from build123d import *

# Parameters (mm, degrees)
SKETCH_1_R          = 21.5
EXTRUDE_1_DEPTH     = 10
EXTRUDE_2_DEPTH     = 5
EXTRUDE_3_DEPTH     = 5
FILLET_1_R          = 10
SKETCH_4_R          = 25
CUT_EXTRUDE_1_DEPTH = 110.56761611
SKETCH_5_R          = 1.65
CUT_EXTRUDE_2_DEPTH = 110.56761611
SKETCH_6_R          = 2.15
CUT_EXTRUDE_3_DEPTH = 92.256849058


with BuildPart() as part:
    # ｽｹｯﾁ1 → ﾎﾞｽ - 押し出し1 (new body)
    with BuildSketch(Plane.XY):
        Circle(SKETCH_1_R)
    extrude(amount=EXTRUDE_1_DEPTH)

    # ｽｹｯﾁ2 → ﾎﾞｽ - 押し出し2 (add)
    with BuildSketch(Plane.XY.offset(10)):
        with BuildLine():
            Line((-21.5, 0), (-21.5, -25))
            Line((-21.5, -25), (21.5, -25))
            Line((21.5, -25), (21.5, 0))
            ThreePointArc((21.5, 0), (0, 21.5), (-21.5, 0))
        make_face()
    extrude(amount=EXTRUDE_2_DEPTH)

    # ｽｹｯﾁ3 → ﾎﾞｽ - 押し出し3 (add)
    with BuildSketch(Plane.XZ.offset(25)):
        with BuildLine():
            Line((-39.25, 54.25), (-39.25, 15))
            Line((-39.25, 15), (39.25, 15))
            Line((39.25, 15), (39.25, 54.25))
            ThreePointArc((39.25, 54.25), (0, 93.5), (-39.25, 54.25))
        make_face()
    extrude(amount=-EXTRUDE_3_DEPTH)

    # ﾌｨﾚｯﾄ1
    fillet_1_edges = [part.edges().sort_by_distance(p)[0] for p in [
        (39.25, -22.5, 15),
        (-39.25, -22.5, 15),
    ]]
    fillet(fillet_1_edges, radius=FILLET_1_R)

    # ｽｹｯﾁ4 → ｶｯﾄ - 押し出し1 (cut, through all)
    with BuildSketch(Plane(origin=(0, -20, 0), x_dir=(1, 0, 0), z_dir=(0, 1, 0))):
        with Locations(Location((0, -54.25, 0), (0, 0, 270))):
            Circle(SKETCH_4_R)
    extrude(amount=-CUT_EXTRUDE_1_DEPTH, mode=Mode.SUBTRACT)

    # ｽｹｯﾁ5 → ｶｯﾄ - 押し出し2 (cut, through all)
    with BuildSketch(Plane(origin=(0, -20, 0), x_dir=(1, 0, 0), z_dir=(0, 1, 0))):
        with Locations(Location((0, -90.75, 0), (0, 0, 270))):
            Circle(SKETCH_5_R)
        with Locations(Location((-23.461747754, -82.210622174, 0), (0, 0, 270))):
            Circle(SKETCH_5_R)
        with Locations(Location((-35.945482985, -60.588158485, 0), (0, 0, 270))):
            Circle(SKETCH_5_R)
        with Locations(Location((-31.609927238, -36, 0), (0, 0, 270))):
            Circle(SKETCH_5_R)
        with Locations(Location((-12.483735231, -19.951219341, 0), (0, 0, 270))):
            Circle(SKETCH_5_R)
        with Locations(Location((12.483735231, -19.951219341, 0), (0, 0, 270))):
            Circle(SKETCH_5_R)
        with Locations(Location((31.609927238, -36, 0), (0, 0, 270))):
            Circle(SKETCH_5_R)
        with Locations(Location((35.945482985, -60.588158485, 0), (0, 0, 270))):
            Circle(SKETCH_5_R)
        with Locations(Location((23.461747754, -82.210622174, 0), (0, 0, 270))):
            Circle(SKETCH_5_R)
    extrude(amount=-CUT_EXTRUDE_2_DEPTH, mode=Mode.SUBTRACT)

    # ｽｹｯﾁ6 → ｶｯﾄ - 押し出し3 (cut, through all)
    with BuildSketch(Plane.XY.offset(15)):
        with Locations((0, 12)):
            Circle(SKETCH_6_R)
        with Locations((10.392304845, 6)):
            Circle(SKETCH_6_R)
        with Locations((10.392304845, -6)):
            Circle(SKETCH_6_R)
        with Locations((0, -12)):
            Circle(SKETCH_6_R)
        with Locations((-10.392304845, -6)):
            Circle(SKETCH_6_R)
        with Locations((-10.392304845, 6)):
            Circle(SKETCH_6_R)
    extrude(amount=-CUT_EXTRUDE_3_DEPTH, mode=Mode.SUBTRACT)


solid = part.part
For this review, take the finished solid that the model builds, in its own axes (mm). A direction names the side the tool comes from. Give positions to 0.01 mm unless a question says otherwise; leave off trailing zeros. Loops run counter-clockwise (first coordinate to the right, second up) from the corner with the lowest first, then second, coordinate; pieces in that order, holes last. Notation, with made-up numbers: M 8,27.5 L 38,27.5 A9 cw 38,35.5 Z; hole C -19.5,22 d7. An arc over 180 degrees is marked long. Answer as a JSON object with one key per item and string values. Group by question number.
Q1. Add section D-D on y = 6. Give the boundary of the cut face in (x, z).
Q2. Add section A-A on x = 0. Give the boundary of the cut face in (y, z).
Q3. For probe 1 along Y at (x, z) = (0, 8.75); probe 2 along Y at (x, z) = (0, 10.5); probe 3 along X at (y, z) = (6.5, 14), list the stretches that pass through material, from the lowest coordinate up. Write a range as [from, to].
Q4. Add section C-C on z = 52. Give the boundary of the cut face in (x, y), and give its area (3 significant figures).
Q5. Insertion check: P1, Ø2, axis at x = 12.48, z = 19.95, coming from the +Y side; P2, Ø8, axis at x = 1, y = 14.5, coming from the +Z side; P3, Ø4.5, axis at x = -35.95, z = 60.59, coming from the +Y side; P4, Ø5.5, axis at y = -15, z = 12, coming from the +X side. Each pin has a flat end and moves straight along its axis. Give the tip position at first contact, or say it passes through.
Q6. Tool access review of faces 4 (the flat face through (0, -22, 10)), 5 (the flat face through (39.25, -23, 39)), 6 (the flat face through (0, 0, 0)), 7 (the flat face through (0, 1, 15)), 8 (the flat face through (-21.5, -12, 12)): name each direction out of +Z, -Z, +X, -X, +Y, -Y from which nothing blocks a thin tool from reaching the whole face with its end or side.
Q7. Mouldability with a two-part tool opening along X and no side actions: class faces 1 (the flat face through (-39.25, -23, 40)), 2 (the cylindrical face through (31.68, -22.46, 34.35)), 3 (the cylindrical face through (36.4, -22.46, 18.01)) as +X half, -X half, draft (parallel to the pull), parting line (faces both ways), or undercut.
Q8. Add section B-B on x = -20. Give the boundary of the cut face in (y, z), and give its area (3 significant figures).
Checked values:
{
 "1": {"outline": "M -20.65,0 L -12.54,0 L -12.54,15 L -20.65,15 Z; M -8.24,0 L 8.24,0 L 8.24,15 L -8.24,15 Z; M 12.54,0 L 20.65,0 L 20.65,15 L 12.54,15 Z"},
 "2": {"outline": "M -25,10 L -21.5,10 L -21.5,0 L -14.15,0 L -14.15,15 L -20,15 L -20,29.25 L -25,29.25 Z; M -25,79.25 L -20,79.25 L -20,89.1 L -25,89.1 Z; M -25,92.4 L -20,92.4 L -20,93.5 L -25,93.5 Z; M -9.85,0 L 9.85,0 L 9.85,15 L -9.85,15 Z; M 14.15,0 L 21.5,0 L 21.5,15 L 14.15,15 Z"},
 "3": {"probe 1": "[-21.5, -14.15], [-9.85, 9.85], [14.15, 21.5]", "probe 2": "[-25, -14.15], [-9.85, 9.85], [14.15, 21.5]", "probe 3": "[-20.49, -12.48], [-8.3, 8.3], [12.48, 20.49]"},
 "4": {"outline": "M -39.25,-25 L -24.9,-25 L -24.9,-20 L -39.25,-20 Z; M 24.9,-25 L 39.25,-25 L 39.25,-20 L 24.9,-20 Z", "area": "144 mm²"},
 "5": {"P1": "through", "P2": "z = 15", "P3": "y = -20", "P4": "x = 21.5"},
 "6": {"face 4": "-Z, -Y", "face 5": "+Z, -Z, +X, +Y, -Y", "face 6": "-Z, +X, -X, +Y, -Y", "face 7": "+Z, +X, -X, +Y", "face 8": "-Z, -X, +Y, -Y"},
 "7": {"face 1": "-X half", "face 2": "undercut", "face 3": "+X half"},
 "8": {"outline": "M -25,10 L -7.89,10 L -7.89,0 L 7.89,0 L 7.89,15 L -20,15 L -20,39.25 L -25,39.25 Z; M -25,69.25 L -20,69.25 L -20,88.02 L -25,88.02 Z", "area": "537 mm²"}
}
